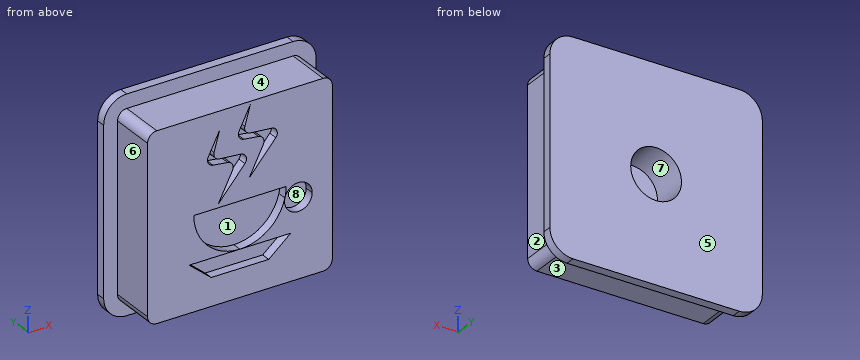
Autodesk Inventor part; units mm, degrees
ref_plane "YZ Plane" through (0, 0, 0) normal (1, 0, 0) x (0, 1, 0)
ref_plane "XZ Plane" through (0, 0, 0) normal (0, 1, 0) x (-1, 0, 0)
ref_plane "XY Plane" through (0, 0, 0) normal (0, 0, 1) x (1, 0, 0)
sketch "Sketch1" plane through (0, 0, 0) normal (0, 1, 0) x (-1, 0, 0)
  line L0 (9, -10) -> (-9, -10)
  line L1 (-10, -9) -> (-10, 9)
  line L2 (-9, 10) -> (9, 10)
  line L3 (10, 9) -> (10, -9)
  line L4 (10, 10) -> (-10, -10) construction
  line L5 (10, -10) -> (-10, 10) construction
  arc A0 (10, 9) -> (9, 10) centre (9, 9) ccw
  arc A1 (9, -10) -> (10, -9) centre (9, -9) ccw
  arc A2 (-10, -9) -> (-9, -10) centre (-9, -9) ccw
  arc A3 (-9, 10) -> (-10, 9) centre (-9, 9) ccw
  point P0 (0, 0)
  point P1 (0, 0)
  dimension "d7" = 20
  dimension "d9" = 20
  dimension "d10" = 1
extrude "Extrusion1" add sketch "Sketch1" along normal blind 5
sketch "Sketch2" plane through (0, 5, 0) normal (0, 1, 0) x (1, 0, 0)
  line L0 (-10, 9) -> (-10, -9)
  arc A0 (-10, -9) -> (-9, -10) centre (-9, -9) ccw
  line L1 (-9, -10) -> (9, -10)
  arc A1 (9, -10) -> (10, -9) centre (9, -9) ccw
  line L2 (10, -9) -> (10, 9)
  arc A2 (10, 9) -> (9, 10) centre (9, 9) ccw
  line L3 (9, 10) -> (-9, 10)
  arc A3 (-9, 10) -> (-10, 9) centre (-9, 9) ccw
  line L4 (9, -11.5) -> (-9, -11.5)
  arc A4 (-11.5, -9) -> (-9, -11.5) centre (-9, -9) ccw
  line L5 (-11.5, -9) -> (-11.5, 9)
  arc A5 (-9, 11.5) -> (-11.5, 9) centre (-9, 9) ccw
  line L6 (-9, 11.5) -> (9, 11.5)
  arc A6 (11.5, 9) -> (9, 11.5) centre (9, 9) ccw
  line L7 (11.5, 9) -> (11.5, -9)
  arc A7 (9, -11.5) -> (11.5, -9) centre (9, -9) ccw
  circle A8 centre (0, 0) radius 2.75
  dimension "d16" = 1.5
  dimension "d19" = 5.5
extrude "Extrusion3" add sketch "Sketch2" along normal blind 1 contours A3 L3 A2 L2 A1 L1 A0 L0 | L4 A4 L5 A5 L6 A6 L7 A7
sketch "Sketch3" plane through (0, 0, 0) normal (0, -1, 0) x (1, 0, 0)
  line L0 (-3.1165, -7) -> (3.1165, -7)
  line L1 (3.1165, -7) -> (5.5, -5)
  line L2 (5.5, -5) -> (-5.5, -5)
  line L3 (-5.5, -5) -> (-3.1165, -7)
  line L4 (0, 0) -> (0, -4.6532) construction
  arc A0 (-5, 0) -> (5, 0) centre (0, 0) ccw
  circle A1 centre (6.3246, -1.5) radius 1.5
  line L5 (-5, 0) -> (5, 0)
  line L6 (-2.2003, 8.0155) -> (-3.4413, 5.57)
  line L7 (-2.9242, 4.5949) -> (-1.3286, 4.3927)
  line L8 (-0.8115, 3.4176) -> (-2.3458, 0.3942)
  line L9 (-2.2003, 8.0155) -> (-2.8111, 5.8955)
  line L10 (-2.2229, 5.0363) -> (0.0906, 4.8285)
  line L11 (0.5397, 3.7134) -> (-2.3458, 0.3942)
  arc A2 (-2.8111, 5.8955) -> (-2.2229, 5.0363) centre (-2.1625, 5.7086) ccw
  arc A3 (0.5397, 3.7134) -> (0.0906, 4.8285) centre (0.0303, 4.1562) ccw
  arc A4 (-0.8115, 3.4176) -> (-1.3286, 4.3927) centre (-1.4135, 3.723) ccw
  arc A5 (-3.4413, 5.57) -> (-2.9242, 4.5949) centre (-2.8393, 5.2646) ccw
  line L12 (1.1412, 9.7016) -> (-0.0998, 7.2561)
  line L13 (0.4173, 6.281) -> (2.0129, 6.0788)
  line L14 (2.53, 5.1037) -> (0.9957, 2.0803)
  line L15 (1.1412, 9.7016) -> (0.5304, 7.5816)
  line L16 (1.1186, 6.7224) -> (3.4321, 6.5146)
  line L17 (3.8812, 5.3995) -> (0.9957, 2.0803)
  arc A6 (0.5304, 7.5816) -> (1.1186, 6.7224) centre (1.179, 7.3947) ccw
  arc A7 (3.8812, 5.3995) -> (3.4321, 6.5146) centre (3.3717, 5.8423) ccw
  arc A8 (2.53, 5.1037) -> (2.0129, 6.0788) centre (1.928, 5.4091) ccw
  arc A9 (-0.0998, 7.2561) -> (0.4173, 6.281) centre (0.5022, 6.9507) ccw
  point P0 (0, -7)
  point P1 (0, -5)
  dimension "d68" = 10
  dimension "d69" = 11
  dimension "d70" = 2
  dimension "d71" = 100
  dimension "d72" = 3
  dimension "d73" = 0.675
  dimension "d74" = 0.675
extrude "Extrusion7" cut sketch "Sketch3" against normal blind 1
hole "Hole1" at (0, 5, 0) direction (0, -1, 0) diameter 5.5 depth 3
equation "\"d7\" = button_side"
equation "\"d9\" = d7"
equation "\"d68\" = 0.5 * button_side"
equation "\"d69\" = 1.1 * d68"
equation "\"d70\" = 0.2 * d68"
equation "\"d72\" = 0.3 * d68"
equation "\"d0\" = 122"
equation "\"d1\" = 77"
equation "\"d4\" = 19"
equation "\"d5\" = 1"
equation "\"d8\" = 25"
equation "\"d13\" = 1.5"
equation "\"d14\" = 0"
equation "\"d15\" = 2"
equation "\"d30\" = 3.1"
equation "\"d31\" = 3"
equation "\"d33\" = 3"
equation "\"d34\" = 2"
equation "\"d36\" = 3"
equation "\"d38\" = 90deg"
equation "\"d39\" = 8"
equation "\"d40\" = 118deg"
equation "\"d44\" = 0"
equation "\"d45\" = 1.2"
equation "\"d46\" = 2"
equation "\"d47\" = 0"
equation "\"d50\" = 25"
equation "\"button_side\" = 20"
equation "\"d3\" = 1.01 * button_side"
equation "\"d2\" = d3"
properties part number "button3" material "Bronze, Soft Tin"
Work out the finished part from the listing and answer in its coordinate system (mm). Face numbers are marked on the shaded views. A direction names the side the tool comes from. Give positions to 0.01 mm unless a question says otherwise; leave off trailing zeros. Loops run counter-clockwise (first coordinate to the right, second up) from the corner with the lowest first, then second, coordinate; pieces in that order, holes last. Notation, with made-up numbers: (58, 41) -> (62, 41) arc R30 cw to (62, 68) -> close; hole circle Ø10 at (77.25, 79). An arc over 180 degrees is marked (long way). Write item = value, one per line. Start each with the question number.
(1) Find the intervals of material crossed by probe 1 along Z at (x, y) = (-3.75, 4.9); probe 2 along Y at (x, z) = (0, 7); probe 3 along Y at (x, z) = (10.75, -1.75), in increasing order. Write a range as from..to.
(2) Find section B-B on x = 6.75. Give the vertices of the cut face in (y, z).
(3) Which of the six approach directions +Z, -Z, +X, -X, +Y, -Y give full straight-line access (tool end or side, diameter ignored) to the marked faces 4, 5, 6, 7 and 8?
(4) Find section C-C on z = -2. Give the vertices of the cut face in (x, y), and give its area (3 significant figures).
(5) Given pin 1 Ø1.5 at (x, z) = (6, -2) entering from -Y; pin 2 Ø0.5 at (x, y) = (-4, 0.5) entering from -Z; pin 3 Ø2.5 at (x, y) = (1, 1.5) entering from +Z, each flat-ended and moving along its own axis, determine where each tip first touches the part or whether it passes through.
(6) The mould has two halves that part along Z. Classify the marked faces 1, 2 and 3: +Z half, -Z half, draft (parallel to the pull), parting line (faces both ways), or undercut.
(7) Find section A-A on y = 4.7. Give the vertices of the cut face in (x, z), and give its area (3 significant figures).
From the geometry:
q1.probe_1 = -10..10
q1.probe_2 = 1..6
q1.probe_3 = 5..6
q2.outline = (0, -10) -> (5, -10) -> (5, -11.5) -> (6, -11.5) -> (6, 11.5) -> (5, 11.5) -> (5, 10) -> (0, 10) -> (0, -0.06) -> (1, -0.06) -> (1, -2.94) -> (0, -2.94) -> close
q3.face_4 = +Z, +X, -X, -Y
q3.face_5 = +Z, -Z, +X, -X, +Y
q3.face_6 = +Z, -Z, -X, -Y
q3.face_7 = +Y
q3.face_8 = -Y
q4.outline = (-11.5, 5) -> (-10, 5) -> (-10, 0) -> (-4.58, 0) -> (-4.58, 1) -> (4.58, 1) -> (4.58, 0) -> (4.91, 0) -> (4.91, 1) -> (7.74, 1) -> (7.74, 0) -> (10, 0) -> (10, 5) -> (11.5, 5) -> (11.5, 6) -> (1.89, 6) -> (1.89, 2) -> (-1.89, 2) -> (-1.89, 6) -> (-11.5, 6) -> close
q4.area = 95.9 mm^2
q5.pin_1 = 1
q5.pin_2 = -10
q5.pin_3 = 10
q6.face_1 = undercut
q6.face_2 = draft
q6.face_3 = -Z half
q7.outline = (-10, -9) arc R1 ccw to (-9, -10) -> (9, -10) arc R1 ccw to (10, -9) -> (10, 9) arc R1 ccw to (9, 10) -> (-9, 10) arc R1 ccw to (-10, 9) -> close; hole circle Ø5.5 at (0, 0)
q7.area = 375 mm^2
